Verification items for the finished model (mm, model axes). A direction names the side the tool comes from. Give positions to 0.01 mm unless a question says otherwise; leave off trailing zeros. Loops run counter-clockwise (first coordinate to the right, second up) from the corner with the lowest first, then second, coordinate; pieces in that order, holes last. Notation, with made-up numbers: M 53.25,-10 L 104.25,-10 A5 ccw 104.25,-2 Z; hole C 12.5,-19 d5. An arc over 180 degrees is marked long. Answer in a Markdown table with one row per item.
```python
from build123d import *

# Parameters (mm, degrees)
SKETCH3_R           = 305
SKETCH3_R_2         = 300
SKETCH3_R_3         = 65
SKETCH3_R_4         = 60
BOSS_EXTRUDE1_DEPTH = 700
BOSS_EXTRUDE2_START = 5
SKETCH4_R           = 305
BOSS_EXTRUDE2_DEPTH = 5
BOSS_EXTRUDE3_START = -5
SKETCH5_R           = 60
BOSS_EXTRUDE3_DEPTH = 5


with BuildPart() as part:
    # Sketch3 → Boss-Extrude1 (new body)
    # profile 1 of 7: a face of its own
    with BuildSketch(Plane(origin=(0, 0, 0), x_dir=(1, 0, 0), z_dir=(0, 1, 0))):
        with Locations(Location((0, 0, 0), (0, 0, 270))):
            Circle(SKETCH3_R)
        Circle(SKETCH3_R_2, mode=Mode.SUBTRACT)
    # profile 2 of 7: a face of its own
    with BuildSketch(Plane(origin=(0, 0, 0), x_dir=(1, 0, 0), z_dir=(0, 1, 0))):
        with BuildLine():
            Line((184.327754195, -236.692372149), (45.841361304, -46.082204741))
            ThreePointArc((45.841361304, -46.082204741), (42.149337524, -49.48164656), (38.206041399, -52.586104634))
            Line((38.206041399, -52.586104634), (176.335575688, -242.705098312))
            ThreePointArc((176.335575688, -242.705098312), (180.356723189, -239.732042915), (184.327754195, -236.692372149))
        make_face()
    # profile 3 of 7: a face of its own
    with BuildSketch(Plane(origin=(0, 0, 0), x_dir=(1, 0, 0), z_dir=(0, 1, 0))):
        with BuildLine():
            Line((282.068231471, 102.164146329), (57.992540793, 29.35754098))
            ThreePointArc((57.992540793, 29.35754098), (60.084703994, 24.795732413), (61.818673559, 20.086104634))
            Line((61.818673559, 20.086104634), (285.316954889, 92.705098312))
            ThreePointArc((285.316954889, 92.705098312), (283.732014095, 97.44816149), (282.068231471, 102.164146329))
        make_face()
    # profile 4 of 7: a face of its own
    with BuildSketch(Plane(origin=(0, 0, 0), x_dir=(1, 0, 0), z_dir=(0, 1, 0))):
        with BuildLine():
            ThreePointArc((-29.661021416, -57.837909787), (-34.034980801, -55.377071807), (-38.206041399, -52.586104634))
            Line((-38.206041399, -52.586104634), (-176.335575688, -242.705098312))
            ThreePointArc((-176.335575688, -242.705098312), (-172.265429064, -245.610712204), (-168.147414308, -248.448077194))
            Line((-168.147414308, -248.448077194), (-29.661021416, -57.837909787))
        make_face()
    # profile 5 of 7: a face of its own
    with BuildSketch(Plane(origin=(0, 0, 0), x_dir=(1, 0, 0), z_dir=(0, 1, 0))):
        Circle(SKETCH3_R_3)
        with Locations(Location((0, 0, 0), (0, 0, 270))):
            Circle(SKETCH3_R_4, mode=Mode.SUBTRACT)
    # profile 6 of 7: a face of its own
    with BuildSketch(Plane(origin=(0, 0, 0), x_dir=(1, 0, 0), z_dir=(0, 1, 0))):
        with BuildLine():
            ThreePointArc((-64.17288068, 10.336410655), (-63.184112466, 15.256733986), (-61.818673559, 20.086104634))
            Line((-61.818673559, 20.086104634), (-285.316954889, 92.705098312))
            ThreePointArc((-285.316954889, 92.705098312), (-286.822613438, 87.936274772), (-288.248571358, 83.143016003))
            Line((-288.248571358, 83.143016003), (-64.17288068, 10.336410655))
        make_face()
    # profile 7 of 7: a face of its own
    with BuildSketch(Plane(origin=(0, 0, 0), x_dir=(1, 0, 0), z_dir=(0, 1, 0))):
        with BuildLine():
            ThreePointArc((-10, 64.226162893), (-5.014948252, 64.806251967), (0, 65))
            Line((0, 65), (0, 300))
            ThreePointArc((0, 300), (-5.000694782, 299.958318857), (-10, 299.833287011))
            Line((-10, 299.833287011), (-10, 64.226162893))
        make_face()
    extrude(amount=BOSS_EXTRUDE1_DEPTH)

    # Sketch4 → Boss-Extrude2 (add)
    with BuildSketch(Plane.XZ.offset(BOSS_EXTRUDE2_START)):
        with Locations(Location((0, 0, 0), (0, 0, 270))):
            Circle(SKETCH4_R)
    extrude(amount=-BOSS_EXTRUDE2_DEPTH)

    # Sketch5 → Boss-Extrude3 (add)
    with BuildSketch(Plane(origin=(0, 700, 0), x_dir=(1, 0, 0), z_dir=(0, 1, 0)).offset(BOSS_EXTRUDE3_START)):
        with Locations(Location((0, 0, 0), (0, 0, 270))):
            Circle(SKETCH5_R)
    extrude(amount=BOSS_EXTRUDE3_DEPTH)


solid = part.part
```
Item 1: Sectioned sample at D-D (z = 96). Record the cut outline in (x, y).
Reported:
| item | result |
|---|---|
| outline | M -289.5,-5 L 289.5,-5 L 289.5,700 L 284.23,700 L 284.23,0 L 82.11,0 L 82.11,700 L 69.75,700 L 69.75,0 L -57.39,0 L -57.39,700 L -69.75,700 L -69.75,0 L -284.23,0 L -284.23,700 L -289.5,700 Z |
Item 2: Sectioned sample at C-C (x = 197). Record the cut outline in (y, z).
Reported:
| item | result |
|---|---|
| outline | M -5,-232.84 L 700,-232.84 L 700,-226.25 L 0,-226.25 L 0,-74.52 L 700,-74.52 L 700,-64.01 L 0,-64.01 L 0,226.25 L 700,226.25 L 700,232.84 L -5,232.84 Z |
Item 3: Scan lines: L1, parallel to X at y = 522, z = 0; L2, parallel to Z at x = 3, y = 66.5 (3 decimals); L3, parallel to Y at x = 0, z = 25. Record each from-to range of solid material in increasing order. Write a range as [from, to].
Reported:
| item | result |
|---|---|
| L1 | x = [-305, -300], [-65, -60], [60, 65], [300, 305] |
| L2 | z = [-304.985, -299.985], [-64.931, -59.925], [59.925, 64.931], [299.985, 304.985] |
| L3 | y = [-5, 0], [695, 700] |
Item 4: Sectioned sample at B-B (z = 0). Record the cut outline in (x, y), and give its area (4 significant figures).
Reported:
| item | result |
|---|---|
| outline | M -305,-5 L 305,-5 L 305,700 L 300,700 L 300,0 L 65,0 L 65,700 L -65,700 L -65,0 L -300,0 L -300,700 L -305,700 Z; hole M -60,0 L 60,0 L 60,695 L -60,695 Z |
| area | 17,650 mm^2 |
Item 5: Tool access check on faces 1 (the cylindrical face through (2.64, 342.64, -59.94)), 2 (the flat face through (1, 700, 21)), 3 (the cylindrical face through (174.4, 345.1, -244.1)). Record the directions out of +Z, -Z, +X, -X, +Y, -Y that give a thin tool (end or side, any length) a straight path to the whole face; none if there is none.
Reported:
| item | result |
|---|---|
| face 1 | none |
| face 2 | +Z, -Z, +X, -X, +Y |
| face 3 | +Y |
Item 6: Go/stop test with flat-tipped pins: pin 1 (12 mm diameter, centred on x = 46, y = 413.5, fed in from -Z); pin 2 (1.5 mm diameter, centred on x = 43.5, y = 326, fed in from -Z); pin 3 (10 mm diameter, centred on x = -204, y = 248.5, fed in from -Z). Record where each tip stops, or that it passes through.
Reported:
| item | result |
|---|---|
| pin 1 | stops at z = -302.37 |
| pin 2 | stops at z = -301.99 |
| pin 3 | stops at z = -231.14 |
Item 7: Release check for a two-part mould opening along X. For faces 4 (the flat face through (112, 0, -163)), 5 (the flat face through (171.6, 345.1, -66.27)), 6 (the flat face through (4, -5, 4)) record: released by +X, released by -X, zero draft, split by the parting line, or undercut.
Reported:
| item | result |
|---|---|
| face 4 | undercut |
| face 5 | undercut |
| face 6 | zero draft |
Item 8: Sectioned sample at A-A (y = 653.5). Record the cut outline in (x, z).
Reported:
| item | result |
|---|---|
| outline | C 0,0 d610; hole M -288.25,-83.14 L -64.17,-10.34 A65 cw -38.21,52.59 L -176.34,242.71 A300 ccw Z; hole M -285.32,-92.71 A300 ccw -10,-299.83 L -10,-64.23 A65 cw -61.82,-20.09 Z; hole M -168.15,248.45 L -29.66,57.84 A65 cw 38.21,52.59 L 176.34,242.71 A300 ccw Z; hole C 0,0 d120; hole M 0,-300 A300 ccw 282.07,-102.16 L 57.99,-29.36 A65 cw 0,-65 Z; hole M 45.84,46.08 A65 cw 61.82,-20.09 L 285.32,-92.71 A300 ccw 184.33,236.69 Z |
